Geometry check sheet. Reference: the model listing, model coordinates, mm. A direction names the side the tool comes from. Round coordinates to 2 decimals unless told otherwise and drop trailing zeros. Write each loop counter-clockwise with the first axis right and the second up, starting at its lowest first coordinate (ties: lowest second). Pieces come first, ordered by that corner, then holes. Notation, with made-up numbers: (-32, 28) -> (-21, 28) arc R21 cw to (-21, 39) -> close; hole circle Ø6 at (58.25, -2.75). An arc over 180 degrees is marked (long way). One line per question, with ' | ' between items.
```python
from build123d import *

# Parameters (mm, degrees)
SKETCH_1_W          = 23.4
SKETCH_1_H          = 12
SKETCH_1_R          = 2.05
SKETCH_1_R_2        = 0.65
SKETCH_1_R_3        = 2.6
EXTRUDE_1_DEPTH     = 1.7
SKETCH_3_R          = 0.65
SKETCH_3_R_2        = 2.6
EXTRUDE_3_DEPTH     = 1.8
EXTRUDE_START       = 1.8
SKETCH_3_16_R       = 2.6
EXTRUDE_4_DEPTH     = 1.8
CUT_EXTRUDE_START   = 5.3
SKETCH_5_R          = 0.8
CUT_EXTRUDE_1_DEPTH = 33.126293072
SKETCH_5_10_R       = 1.5
CUT_EXTRUDE_3_DEPTH = 3.3
SKETCH_7_R          = 0.35
CUT_EXTRUDE_4_DEPTH = 2


with BuildPart() as part:
    # 草图1 → 凸台-拉伸1 (new body)
    with BuildSketch(Plane(origin=(0, 0, 0), x_dir=(1, 0, 0), z_dir=(0, 1, 0))):
        with Locations((11.7, -6)):
            Rectangle(SKETCH_1_W, SKETCH_1_H)
        with Locations(Location((5, -6, 0), (0, 0, 270))):
            Circle(SKETCH_1_R, mode=Mode.SUBTRACT)
        with Locations(Location((9.270831301, -8.6, 0), (0, 0, 270))):
            Circle(SKETCH_1_R_2, mode=Mode.SUBTRACT)
        with Locations(Location((18.395740059, -6, 0), (0, 0, 270))):
            Circle(SKETCH_1_R_3, mode=Mode.SUBTRACT)
        with Locations(Location((9.270831301, -3.4, 0), (0, 0, 270))):
            Circle(SKETCH_1_R_2, mode=Mode.SUBTRACT)
    extrude(amount=EXTRUDE_1_DEPTH)

    # 草图3 → 凸台-拉伸3 (add)
    with BuildSketch(Plane(origin=(0, 1.7, 0), x_dir=(1, 0, 0), z_dir=(0, 1, 0))):
        with BuildLine():
            Line((6.322950706, 0), (0, 0))
            Line((0, 0), (0, -12))
            Line((0, -12), (23.4, -12))
            Line((23.4, -12), (23.4, 0))
            Line((23.4, 0), (12.218711895, 0))
            ThreePointArc((12.218711895, 0), (12.831329536, -6.151881595), (6.723669831, -7.109712717))
            ThreePointArc((6.723669831, -7.109712717), (3.248959167, -7.066), (4.805714858, -3.959227283))
            ThreePointArc((4.805714858, -3.959227283), (5.068807808, -1.789720968), (6.322950706, 0))
        make_face()
        with Locations(Location((9.270831301, -8.6, 0), (0, 0, 270))):
            Circle(SKETCH_3_R, mode=Mode.SUBTRACT)
        with Locations(Location((18.395740059, -6, 0), (0, 0, 270))):
            Circle(SKETCH_3_R_2, mode=Mode.SUBTRACT)
    extrude(amount=EXTRUDE_3_DEPTH)

    # 草图3<16> → 凸台-拉伸4 (add)
    # profile 1 of 2: a face of its own
    with BuildSketch(Plane(origin=(0, 1.7, 0), x_dir=(1, 0, 0), z_dir=(0, 1, 0)).offset(EXTRUDE_START)):
        with BuildLine():
            Line((6.322950706, 0), (0, 0))
            Line((0, 0), (0, -12))
            Line((0, -12), (6.322950706, -12))
            ThreePointArc((6.322950706, -12), (5.068807808, -10.210279032), (4.805714858, -8.040772717))
            ThreePointArc((4.805714858, -8.040772717), (2.95, -6), (4.805714858, -3.959227283))
            ThreePointArc((4.805714858, -3.959227283), (5.068807808, -1.789720968), (6.322950706, 0))
        make_face()
    # profile 2 of 2: a face of its own
    with BuildSketch(Plane(origin=(0, 1.7, 0), x_dir=(1, 0, 0), z_dir=(0, 1, 0)).offset(EXTRUDE_START)):
        with BuildLine():
            Line((23.4, 0), (12.218711895, 0))
            ThreePointArc((12.218711895, 0), (13.364452111, -1.531238736), (13.770831301, -3.4))
            ThreePointArc((13.770831301, -3.4), (13.559067005, -4.7641974), (12.943704835, -6))
            ThreePointArc((12.943704835, -6), (13.559067005, -7.2358026), (13.770831301, -8.6))
            ThreePointArc((13.770831301, -8.6), (13.364452111, -10.468761264), (12.218711895, -12))
            Line((12.218711895, -12), (23.4, -12))
            Line((23.4, -12), (23.4, 0))
        make_face()
        with Locations(Location((18.395740059, -6, 0), (0, 0, 270))):
            Circle(SKETCH_3_16_R, mode=Mode.SUBTRACT)
    extrude(amount=EXTRUDE_4_DEPTH)

    # 草图5 → 切除-拉伸1 (cut, through all)
    with BuildSketch(Plane(origin=(0, 0, 0), x_dir=(1, 0, 0), z_dir=(0, 1, 0)).offset(CUT_EXTRUDE_START)):
        with Locations(Location((2.3, -2.214171161, 0), (0, 0, 270))):
            Circle(SKETCH_5_R)
        with Locations(Location((7.7, -9.785828839, 0), (0, 0, 270))):
            Circle(SKETCH_5_R)
    extrude(amount=-CUT_EXTRUDE_1_DEPTH, mode=Mode.SUBTRACT)

    # 草图5<10> → 切除-拉伸3 (cut)
    with BuildSketch(Plane(origin=(0, 0, 0), x_dir=(1, 0, 0), z_dir=(0, 1, 0)).offset(CUT_EXTRUDE_START)):
        with Locations(Location((2.3, -2.214171161, 0), (0, 0, 270))):
            Circle(SKETCH_5_10_R)
        with Locations((7.7, -9.785828839)):
            Circle(SKETCH_5_10_R)
    extrude(amount=-CUT_EXTRUDE_3_DEPTH, mode=Mode.SUBTRACT)

    # 草图7 → 切除-拉伸4 (cut)
    with BuildSketch(Plane(origin=(0, 5.3, 0), x_dir=(1, 0, 0), z_dir=(0, 1, 0))):
        with Locations(Location((1.568943185, -5.332489754, 0), (0, 0, 270))):
            Circle(SKETCH_7_R)
        with Locations(Location((2.419185522, -9.817518082, 0), (0, 0, 270))):
            Circle(SKETCH_7_R)
        with Locations(Location((21.143175994, -2.108925173, 0), (0, 0, 270))):
            Circle(SKETCH_7_R)
        with Locations(Location((21.143175994, -9.817518082, 0), (0, 0, 270))):
            Circle(SKETCH_7_R)
    extrude(amount=-CUT_EXTRUDE_4_DEPTH, mode=Mode.SUBTRACT)


solid = part.part
```
(1) Go/stop test with flat-tipped pins: pin 1 (0.9 mm diameter, centred on x = 7.5, z = 10.5, fed in from +Y); pin 2 (0.8 mm diameter, centred on x = 2.5, z = 10, fed in from +Y); pin 3 (6.5 mm diameter, centred on x = 9, z = 9.5, fed in from +Y). Record where each tip stops, or that it passes through.
Resolved:
pin 1: stops at y = 2 | pin 2: stops at y = 5.3 | pin 3: stops at y = 3.5
(2) Sectioned sample at B-B on y = 3.8. Record the cut outline in (x, z), then the cut area to 3 significant figures.
Resolved:
outline: (0, 0) -> (6.32, 0) arc R4.5 cw to (4.81, 3.96) arc R2.05 cw to (4.81, 8.04) arc R4.5 cw to (6.32, 12) -> (0, 12) -> close; (12.22, 0) -> (23.4, 0) -> (23.4, 12) -> (12.22, 12) arc R4.5 cw to (12.94, 6) arc R4.5 cw to start; hole circle Ø3 at (2.3, 2.21); hole circle Ø0.7 at (1.57, 5.33); hole circle Ø0.7 at (2.42, 9.82); hole circle Ø5.2 at (18.4, 6); hole circle Ø0.7 at (21.14, 2.11); hole circle Ø0.7 at (21.14, 9.82) | area: 145 mm2
(3) Sectioned sample at A-A on z = 4.5. Record the cut outline in (x, y), then the cut area to 3 significant figures.
Resolved:
outline: (0, 0) -> (3.6, 0) -> (3.6, 5.3) -> (0, 5.3) -> close; (6.4, 0) -> (16.27, 0) -> (16.27, 5.3) -> (13.63, 5.3) -> (13.63, 1.7) -> (6.4, 1.7) -> close; (20.52, 0) -> (23.4, 0) -> (23.4, 5.3) -> (20.52, 5.3) -> close | area: 60.6 mm2
(4) Sectioned sample at C-C on x = 7.7. Record the cut outline in (y, z), then the cut area to 3 significant figures.
Resolved:
outline: (0, 0) -> (1.7, 0) -> (1.7, 7.62) -> (3.5, 7.62) -> (3.5, 8.29) -> (2, 8.29) -> (2, 8.99) -> (0, 8.99) -> close; (0, 10.59) -> (2, 10.59) -> (2, 11.29) -> (3.5, 11.29) -> (3.5, 12) -> (0, 12) -> close | area: 20.6 mm2
(5) Access from +Z, -Z, +X, -X, +Y, -Y to the whole of each face (thin tool, end or side, straight path). Record for faces 1 (the cylindrical face through (3.787, 3.673, 2.019)), 2 (the cylindrical face through (2.54, 1.014, 2.977)).
Resolved:
face 1: +Y | face 2: +Y, -Y
(6) Material ranges on line 1 (X direction, y = 2.65, z = 6); line 2 (Z direction, x = 3.25, y = 3.85); line 3 (X direction, y = 3.3, z = 6.75), recorded low to high.
Resolved:
line 1: x = 0 to 2.95, 12.94 to 15.8, 21 to 23.4 | line 2: z = 0 to 1.05, 3.37 to 4.93, 7.07 to 12 | line 3: x = 0 to 3.09, 12.28 to 15.91, 20.89 to 23.4
(7) Draft check along Z on faces 3 (the flat face through (12, 3, 12)), 4 (the flat face through (2, 5.3, 6)), 5 (the cylindrical face through (7.394, 1.014, 10.525)). Enter one of: +Z half, -Z half, draft (parallel to the pull), parting line (faces both ways), or undercut.
Resolved:
face 3: +Z half | face 4: draft | face 5: undercut
(8) Sectioned sample at D-D on y = 1.25. Record the cut outline in (x, z).
Resolved:
outline: (0, 0) -> (23.4, 0) -> (23.4, 12) -> (0, 12) -> close; hole circle Ø1.6 at (2.3, 2.21); hole circle Ø4.1 at (5, 6); hole circle Ø1.6 at (7.7, 9.79); hole circle Ø1.3 at (9.27, 3.4); hole circle Ø1.3 at (9.27, 8.6); hole circle Ø5.2 at (18.4, 6)
